The listing builds one solid part. Answer for the finished solid, in the listing's coordinates (mm). Round coordinates to 2 decimals unless told otherwise and drop trailing zeros. Loops run counter-clockwise (first coordinate to the right, second up) from the corner with the lowest first, then second, coordinate; pieces in that order, holes last. Notation, with made-up numbers: (-24, 34.25) -> (16, 34.25) arc R13 cw to (16, 53.25) -> close; hole circle Ø1 at (26, 29.25). An arc over 180 degrees is marked (long way). Write each question's results on one line, items separated by ' | '. Start each with the question number.
(1) The part is cut by section C-C (y = 0.85). Determine the outline of the cut face in (x, z).
(2) Straight lines are drawn through the part: probe 1 along X at (y, z) = (1.55, 0); probe 2 along Y at (x, z) = (8.75, 2.5); probe 3 along Z at (x, y) = (-2.5, 2.2). For each, find the intervals that lie inside material, in ascending order.
(3) Flat-ended cylindrical pins translate along their axes: pin 1 (3.5 mm diameter, centred on x = 1.5, z = -0.5, fed in from +Y); pin 2 (1 mm diameter, centred on x = -6.5, z = 1, fed in from -Y). Find the tip coordinate at first contact, or state that the pin passes through.
(4) Determine the mould class of faces 1 (the face through (-3.9, 0, -7.3)), 2 (the face through (-3.905, 1.363, -0.867)), 3 (the face through (0, 0.5, 0)), 4 (the face through (-3.417, 1.363, -0.759)) for opening direction X: released by +X, released by -X, zero draft, split by the parting line, or undercut.
```python
from build123d import *

# Parameters (mm, degrees)
SKETCH_1_R      = 11
EXTRUDE_1_DEPTH = 0.5
SKETCH_2_R      = 4
SKETCH_2_R_2    = 3.5
EXTRUDE_2_DEPTH = 2
FILLET_1_R      = 0.25
FILLET_2_R      = 0.2


with BuildPart() as part:
    # 草图1 → 凸台-拉伸1 (new body)
    with BuildSketch(Plane(origin=(0, 0, 0), x_dir=(1, 0, 0), z_dir=(0, 1, 0))):
        with Locations(Location((0, 0, 0), (0, 0, 270))):
            Circle(SKETCH_1_R)
    extrude(amount=EXTRUDE_1_DEPTH)

    # 草图2 → 凸台-拉伸2 (add)
    with BuildSketch(Plane(origin=(0, 0.5, 0), x_dir=(1, 0, 0), z_dir=(0, 1, 0))):
        with Locations(Location((0, 0, 0), (0, 0, 270))):
            Circle(SKETCH_2_R)
        with Locations(Location((0, 0, 0), (0, 0, 270))):
            Circle(SKETCH_2_R_2, mode=Mode.SUBTRACT)
    extrude(amount=EXTRUDE_2_DEPTH)

    # 圆角1
    fillet_1_edges = [part.edges().sort_by_distance(p)[0] for p in [
        (0, 2.5, -4),
        (0, 2.5, -3.5),
    ]]
    fillet(fillet_1_edges, radius=FILLET_1_R - 0.0001)  # a hair under: the kernel refuses the full size

    # 草图3 → 切除-旋转2 (revolve, cut)
    with BuildSketch(Plane(origin=(0, 0, 0), x_dir=(0, 0, -1), z_dir=(1, 0, 0)), mode=Mode.PRIVATE) as cut_revolve_2_sk:
        with BuildLine():
            Line((0, 0), (8, 0))
            ThreePointArc((8, 0), (4.002811512, 0.224973651), (0, 0.3))
            Line((0, 0.3), (0, 0))
        make_face()
    revolve(cut_revolve_2_sk.sketch.rotate(Axis((0, 0, 0), (0, 1, 0)), 180), axis=Axis((0, 0, 0), (0, 1, 0)), mode=Mode.SUBTRACT)

    # 圆角2
    fillet_2_edges = [part.edges().sort_by_distance(p)[0] for p in [
        (0, 0, -11),
        (0, 0.5, -11),
    ]]
    fillet(fillet_2_edges, radius=FILLET_2_R)


solid = part.part
```
Checked values:
1) outline: circle Ø8 at (0, 0); hole circle Ø7 at (0, 0)
2) probe 1: x = -4 to -3.5, 3.5 to 4 | probe 2: y = 0 to 0.5 | probe 3: z = -3.12 to -2.45, 2.45 to 3.12
3) pin 1: stops at y = 0.5 | pin 2: stops at y = 0.07
4) face 1: zero draft | face 2: split by the parting line | face 3: undercut | face 4: undercut
